```python
from build123d import *

# Parameters (mm, degrees)
BOSS_EXTRUDE1_DEPTH = 20
SKETCH2_W           = 60
SKETCH2_H           = 10
CUT_EXTRUDE1_DEPTH  = 182.383571472
SKETCH3_W           = 80
SKETCH3_H           = 100
BOSS_EXTRUDE2_DEPTH = 20
BOSS_EXTRUDE4_DEPTH = 60
CUT_EXTRUDE5_DEPTH  = 189.745860882
SKETCH12_R          = 15
CUT_EXTRUDE6_DEPTH  = 198.230829233
SKETCH13_W          = 60
SKETCH13_H          = 60
CUT_EXTRUDE7_DEPTH  = 10


with BuildPart() as part:
    # Sketch1 → Boss-Extrude1 (new body)
    with BuildSketch(Plane(origin=(0, 0, 0), x_dir=(1, 0, 0), z_dir=(0, 1, 0))):
        with BuildLine():
            Line((135, 58), (150, 58))
            Line((150, 58), (150, 100))
            Line((150, 100), (0, 100))
            Line((0, 100), (0, 58))
            Line((0, 58), (15, 58))
            ThreePointArc((15, 58), (23, 50), (15, 42))
            Line((15, 42), (0, 42))
            Line((0, 42), (0, 0))
            Line((0, 0), (150, 0))
            Line((150, 0), (150, 42))
            Line((150, 42), (135, 42))
            ThreePointArc((135, 42), (127, 50), (135, 58))
        make_face()
    extrude(amount=BOSS_EXTRUDE1_DEPTH)

    # Sketch2 → Cut-Extrude1 (cut, through all)
    with BuildSketch(Plane(origin=(150, 0, 0), x_dir=(0, 0, -1), z_dir=(1, 0, 0))):
        with Locations((50, 5)):
            Rectangle(SKETCH2_W, SKETCH2_H)
    extrude(amount=-CUT_EXTRUDE1_DEPTH, mode=Mode.SUBTRACT)

    # Sketch3 → Boss-Extrude2 (add)
    with BuildSketch(Plane(origin=(0, 20, 0), x_dir=(1, 0, 0), z_dir=(0, 1, 0))):
        with Locations((75, 50)):
            Rectangle(SKETCH3_W, SKETCH3_H)
    extrude(amount=BOSS_EXTRUDE2_DEPTH)

    # Sketch8 → Boss-Extrude4 (add)
    with BuildSketch(Plane(origin=(0, 40, 0), x_dir=(1, 0, 0), z_dir=(0, 1, 0))):
        Polygon((115, 100), (35, 100), (35, 0), (45, 0), (45, 80), (105, 80), (105, 0), (115, 0), align=None)
    extrude(amount=BOSS_EXTRUDE4_DEPTH)

    # Sketch11 → Cut-Extrude5 (cut, through all)
    with BuildSketch(Plane(origin=(125, 0, 0), x_dir=(0, 0, -1), z_dir=(1, 0, 0))):
        Polygon((0, 40), (80, 100), (0, 100), align=None)
    extrude(amount=-CUT_EXTRUDE5_DEPTH, mode=Mode.SUBTRACT)

    # Sketch12 → Cut-Extrude6 (cut, through all)
    with BuildSketch(Plane.XY.offset(-80)):
        with Locations((75, 60)):
            Circle(SKETCH12_R)
    extrude(amount=-CUT_EXTRUDE6_DEPTH, mode=Mode.SUBTRACT)

    # Sketch13 → Cut-Extrude7 (cut)
    with BuildSketch(Plane.XY.offset(-80)):
        with Locations((75, 70)):
            Rectangle(SKETCH13_W, SKETCH13_H)
    extrude(amount=-CUT_EXTRUDE7_DEPTH, mode=Mode.SUBTRACT)


solid = part.part
```
Geometry: final body of the model. Coordinates: model frame, mm. A direction names the side the tool comes from. Coordinates: 2 decimals unless noted, no trailing zeros. Order: outer loops, then holes, each group sorted by start corner. A loop starts at its lowest first (then second) coordinate and runs counter-clockwise, first axis right, second up. Notation, with made-up numbers: (-38, 52.5) - (-1, 52.5) arc R10 cw to (-1, 66.5) - close; hole circle Ø9 at (65.25, -24). An arc over 180 degrees is marked (long way). Write each question's results on one line, items separated by ' | '.
1) Pin query (flat end, axial travel): pin 1 (6 mm diameter, centred on y = 36, z = -50.5, fed in from +X); pin 2 (4 mm diameter, centred on x = 60, z = -25.5, fed in from +Y); pin 3 (1 mm diameter, centred on x = 28.5, z = -72.5, fed in from -Y); pin 4 (24 mm diameter, centred on x = 75, y = 60, fed in from -Z). Return the tip coordinate at first contact, or that it passes through.
Results list:
pin 1: x = 115 | pin 2: y = 40 | pin 3: y = 10 | pin 4: through
2) Pull-direction query (Y, two-part tool) for faces 5 (the cylindrical face through (71.748, 45.357, -94.93)), 6 (the flat face through (76, 10, -50)), 7 (the cylindrical face through (127, 15, -50)); classes: pulls with the +Y half, pulls with the -Y half, needs draft (parallel to the pull), parting line crosses it, or undercut.
Results list:
face 5: undercut | face 6: pulls with the -Y half | face 7: needs draft
3) Section D-D, the plane z = -76. Return loops of the section in (x, y), plus the area to 3 significant figures.
Results list:
outline: (0, 10) - (150, 10) - (150, 20) - (115, 20) - (115, 97) - (105, 97) - (105, 40) - (45, 40) - (45, 97) - (35, 97) - (35, 20) - (0, 20) - close | area: 4,240 mm^2
4) Line query: line 1 (Y direction, x = 75, z = -92); line 2 (Y direction, x = 61, z = -65.5); line 3 (Y direction, x = 131, z = -65). Output: solid intervals per line, ascending. Write a range as from..to.
Results list:
line 1: 0..45, 75..100 | line 2: 10..40 | line 3: 10..20
5) Section B-B, the plane y = 62. Return loops of the section in (x, z), plus the area to 3 significant figures.
Results list:
outline: (35, -100) - (60.13, -100) - (60.13, -90) - (45, -90) - (45, -29.33) - (35, -29.33) - close; (89.87, -100) - (115, -100) - (115, -29.33) - (105, -29.33) - (105, -90) - (89.87, -90) - close | area: 1,720 mm^2
6) Section A-A, the plane x = 75. Return loops of the section in (y, z), plus the area to 3 significant figures.
Results list:
outline: (0, -100) - (45, -100) - (45, -90) - (40, -90) - (40, 0) - (0, 0) - (0, -20) - (10, -20) - (10, -80) - (0, -80) - close; (75, -100) - (100, -100) - (100, -90) - (75, -90) - close | area: 3,700 mm^2
7) Section C-C, the plane x = 117.5. Return loops of the section in (y, z), plus the area to 3 significant figures.
Results list:
outline: (0, -100) - (20, -100) - (20, 0) - (0, 0) - (0, -20) - (10, -20) - (10, -80) - (0, -80) - close | area: 1,400 mm^2
8) Set-up query: faces 1 (the flat face through (76, 5, -20)), 2 (the flat face through (75, 77, -90)), 3 (the flat face through (35, 51, -62)), 4 (the flat face through (8, 15, -42)). Return all of +Z, -Z, +X, -X, +Y, -Y with unobstructed straight access to the full face (end or side cutting, diameter ignored); none if empty.
Results list:
face 1: +X, -X, -Y | face 2: +Z, +Y | face 3: +Z, -Z, -X, +Y | face 4: -X, +Y, -Y
